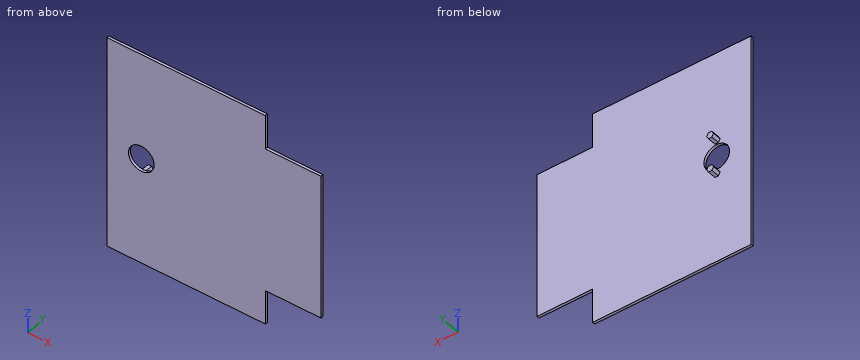
```python
from build123d import *

# Parameters (mm, degrees)
SKETCH1_R           = 15
BOSS_EXTRUDE2_DEPTH = 3
BOSS_EXTRUDE3_DEPTH = 10


with BuildPart() as part:
    # Sketch1 → Boss-Extrude2 (new body)
    with BuildSketch(Plane(origin=(0, 0, 0), x_dir=(1, 0, 0), z_dir=(0, 1, 0))):
        Polygon((0, 0), (185, 0), (185, 40), (250, 40), (250, 210), (185, 210), (185, 250), (0, 250), align=None)
        with Locations(Location((40, 125, 0), (0, 0, 270))):
            Circle(SKETCH1_R, mode=Mode.SUBTRACT)
    extrude(amount=BOSS_EXTRUDE2_DEPTH)

    # Sketch2 → Boss-Extrude3 (add)
    with BuildSketch(Plane(origin=(0, 3, 0), x_dir=(1, 0, 0), z_dir=(0, 1, 0))):
        Polygon((44.041451884, 145), (42.020725942, 148.5), (37.979274058, 148.5), (35.958548116, 145), (37.979274058, 141.5), (42.020725942, 141.5), align=None)
        Polygon((44.041451884, 105), (42.020725942, 108.5), (37.979274058, 108.5), (35.958548116, 105), (37.979274058, 101.5), (42.020725942, 101.5), align=None)
    extrude(amount=BOSS_EXTRUDE3_DEPTH)


solid = part.part
```
Model file for the job. Use its own axes, mm. Give positions to 0.01 mm unless a question says otherwise; leave off trailing zeros. Order: outer loops, then holes, each group sorted by start corner. A loop starts at its lowest first (then second) coordinate and runs counter-clockwise, first axis right, second up.
1) Pin check, flat tips, straight feed: pin 1 (4.5 mm diameter, centred on x = 40, y = 6, fed in from -Z); pin 2 (1.2 mm diameter, centred on x = 39.5, y = 8.5, fed in from +Z); pin 3 (2.5 mm diameter, centred on x = 229, y = 1, fed in from -Z); pin 4 (1.5 mm diameter, centred on x = 31, y = 5.5, fed in from -Z). Stop position of each tip, or through.
2) Wall check: probe 1 along X at (y, z) = (1.25, -125); probe 2 along Y at (x, z) = (174, -76); probe 3 along X at (y, z) = (2.5, -32.5). Give the ranges that are in metal, low to high.
3) Saw through at C-C, the plane x = 167.5. Write the cut outline in (y, z).
4) Saw through at D-D, the plane z = -59. Write the cut outline in (x, y).
5) Saw through at A-A, the plane z = -125. Write the cut outline in (x, y), then the cut area to 3 significant figures.
6) Saw through at B-B, the plane y = 11. Write the cut outline in (x, z), then the cut area to 3 significant figures.
Computed:
1. pin 1: stops at z = -148.5
1. pin 2: stops at z = -101.5
1. pin 3: stops at z = -210
1. pin 4: passes through
2. probe 1: x = 0 to 25, 55 to 250
2. probe 2: y = 0 to 3
2. probe 3: x = 0 to 185
3. outline: (0, -250) - (3, -250) - (3, 0) - (0, 0) - close
4. outline: (0, 0) - (250, 0) - (250, 3) - (0, 3) - close
5. outline: (0, 0) - (25, 0) - (25, 3) - (0, 3) - close; (55, 0) - (250, 0) - (250, 3) - (55, 3) - close
5. area: 660 mm2
6. outline: (35.96, -145) - (37.98, -148.5) - (42.02, -148.5) - (44.04, -145) - (42.02, -141.5) - (37.98, -141.5) - close; (35.96, -105) - (37.98, -108.5) - (42.02, -108.5) - (44.04, -105) - (42.02, -101.5) - (37.98, -101.5) - close
6. area: 84.9 mm2
